from build123d import *

# Parameters (mm, degrees)
SKETCH1_R      = 3
EXTRUDE1_DEPTH = 18
SKETCH1_3_R    = 19.05
EXTRUDE2_DEPTH = 10
SKETCH2_R      = 1.52
EXTRUDE3_DEPTH = 37.59
EXTRUDE4_START = -2.6
SKETCH3_W      = 29.21
SKETCH3_H      = 15
EXTRUDE4_DEPTH = 34.99
EXTRUDE6_DEPTH = 10
SKETCH8_R      = 1.53
EXTRUDE7_DEPTH = 43
EXTRUDE8_DEPTH = 37.59


with BuildPart() as part:
    # Sketch1 → Extrude1 (new body)
    with BuildSketch(Plane(origin=(0, 0, 0), x_dir=(1, 0, 0), z_dir=(0, 1, 0))):
        with BuildLine():
            Line((-10.033035154, 21.134136258), (126.344272034, 21.134136258))
            ThreePointArc((126.344272034, 21.134136258), (129.573902971, 21.670020662), (132.457392138, 23.220239455))
            ThreePointArc((132.457392138, 23.220239455), (166.412495407, 0.194425945), (125.416806741, -1.383749149))
            ThreePointArc((125.416806741, -1.383749149), (121.751361628, 3.344530461), (116.04264662, 5.134136258))
            Line((116.04264662, 5.134136258), (0.26859026, 5.134136258))
            ThreePointArc((0.26859026, 5.134136258), (-5.440124747, 3.344530461), (-9.10556986, -1.383749149))
            ThreePointArc((-9.10556986, -1.383749149), (-50.101258526, 0.194425945), (-16.146155257, 23.220239455))
            ThreePointArc((-16.146155257, 23.220239455), (-13.262666091, 21.670020662), (-10.033035154, 21.134136258))
        make_face()
        with Locations((-29.34438156, 6.134136258)):
            Circle(SKETCH1_R, mode=Mode.SUBTRACT)
        with Locations((145.65561844, 6.134136258)):
            Circle(SKETCH1_R, mode=Mode.SUBTRACT)
    extrude(amount=EXTRUDE1_DEPTH)

    # Sketch1<3> → Extrude2 (cut)
    with BuildSketch(Plane(origin=(0, 0, 0), x_dir=(1, 0, 0), z_dir=(0, 1, 0))):
        with Locations((-29.34438156, 6.134136258)):
            Circle(SKETCH1_3_R)
        with Locations((145.65561844, 6.134136258)):
            Circle(SKETCH1_3_R)
    extrude(amount=EXTRUDE2_DEPTH, mode=Mode.SUBTRACT)

    # Sketch2 → Extrude3 (cut, through all)
    with BuildSketch(Plane(origin=(0, 0, -21.134136258), x_dir=(-1, 0, 0), z_dir=(0, 0, -1))):
        with Locations((-68.542401875, 7.04)):
            Circle(SKETCH2_R)
        with Locations((-47.61061844, 7.04)):
            Circle(SKETCH2_R)
    extrude(amount=-EXTRUDE3_DEPTH, mode=Mode.SUBTRACT)

    # Sketch3 → Extrude4 (cut, through all)
    with BuildSketch(Plane(origin=(0, 0, -21.134136258), x_dir=(-1, 0, 0), z_dir=(0, 0, -1)).offset(EXTRUDE4_START)):
        with Locations((-58.15561844, 7.5)):
            Rectangle(SKETCH3_W, SKETCH3_H)
    extrude(amount=-EXTRUDE4_DEPTH, mode=Mode.SUBTRACT)

    # Sketch6 → Extrude6 (cut)
    with BuildSketch(Plane(origin=(0, 18, 0), x_dir=(1, 0, 0), z_dir=(0, 1, 0))):
        with BuildLine():
            Line((41.01061844, 13.134136258), (41.01061844, 16.546636258))
            ThreePointArc((41.01061844, 16.546636258), (40.545650455, 17.669168273), (39.42311844, 18.134136258))
            Line((39.42311844, 18.134136258), (4.59811844, 18.134136258))
            ThreePointArc((4.59811844, 18.134136258), (3.475586425, 17.669168273), (3.01061844, 16.546636258))
            Line((3.01061844, 16.546636258), (3.01061844, 9.721636258))
            ThreePointArc((3.01061844, 9.721636258), (3.475586425, 8.599104243), (4.59811844, 8.134136258))
            Line((4.59811844, 8.134136258), (39.42311844, 8.134136258))
            ThreePointArc((39.42311844, 8.134136258), (40.545650455, 8.599104243), (41.01061844, 9.721636258))
            Line((41.01061844, 9.721636258), (41.01061844, 13.134136258))
        make_face()
        with BuildLine():
            Line((75.30061844, 9.721636258), (75.30061844, 13.134136258))
            Line((75.30061844, 13.134136258), (75.30061844, 16.546636258))
            ThreePointArc((75.30061844, 16.546636258), (75.765586425, 17.669168273), (76.88811844, 18.134136258))
            Line((76.88811844, 18.134136258), (111.71311844, 18.134136258))
            ThreePointArc((111.71311844, 18.134136258), (112.835650455, 17.669168273), (113.30061844, 16.546636258))
            Line((113.30061844, 16.546636258), (113.30061844, 9.721636258))
            ThreePointArc((113.30061844, 9.721636258), (112.835650455, 8.599104243), (111.71311844, 8.134136258))
            Line((111.71311844, 8.134136258), (76.88811844, 8.134136258))
            ThreePointArc((76.88811844, 8.134136258), (75.765586425, 8.599104243), (75.30061844, 9.721636258))
        make_face()
    extrude(amount=-EXTRUDE6_DEPTH, mode=Mode.SUBTRACT)

    # Sketch8 → Extrude7 (cut)
    with BuildSketch(Plane(origin=(75.30061844, 0, 0), x_dir=(0, 0, -1), z_dir=(1, 0, 0))):
        with Locations((13.696636258, 12.37)):
            Circle(SKETCH8_R)
    extrude(amount=-EXTRUDE7_DEPTH, mode=Mode.SUBTRACT)

    # Sketch9 → Extrude8 (cut, through all)
    with BuildSketch(Plane(origin=(0, 0, -21.134136258), x_dir=(-1, 0, 0), z_dir=(0, 0, -1))):
        with BuildLine():
            ThreePointArc((-68.427924828, 0), (-58.131552552, -10.4619369), (-47.724510158, -0.110083234))
            ThreePointArc((-47.724510158, -0.110083234), (-47.724656491, -0.055040839), (-47.725095487, 0))
            Line((-47.725095487, 0), (-68.427924828, 0))
        make_face()
        with BuildLine():
            Line((-68.427924828, 0), (-47.725095487, 0))
            ThreePointArc((-47.725095487, 0), (-58.076510158, 10.241916766), (-68.427924828, 0))
        make_face()
    extrude(amount=-EXTRUDE8_DEPTH, mode=Mode.SUBTRACT)


solid = part.part
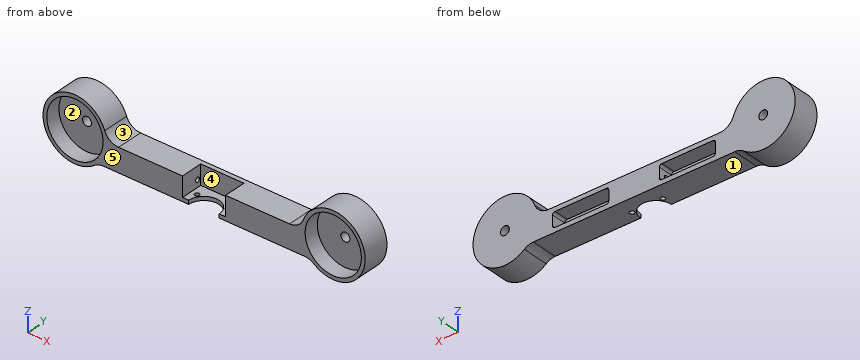
Can you work these out from the model? Positions are in its coordinate system, mm. Face numbers are marked on the shaded views. A direction names the side the tool comes from. Round coordinates to 2 decimals unless told otherwise and drop trailing zeros. Write each loop counter-clockwise with the first axis right and the second up, starting at its lowest first coordinate (ties: lowest second). Pieces come first, ordered by that corner, then holes. Notation, with made-up numbers: (82, 77) -> (124, 77) arc R31 cw to (124, 113) -> close; hole circle Ø3 at (20, 63.25). An arc over 180 degrees is marked (long way). One line per question, with ' | ' between items. Start each with the question number.
1) On a 3-axis mill with a long thin cutter (end or side, diameter ignored), from which of +Z, -Z, +X, -X, +Y, -Y can I reach the whole of each face in a straight line? I mean the marked faces 1, 2 and 3. Say none if no direction works.
2) Suppose I cut it at D-D on x = 58.5. Write out the boundary of the cut face in (y, z).
3) I need wall thicknesses on line 1 (Z direction, x = 102, y = 10.5); line 2 (Z direction, x = 145.5, y = 15.5); line 3 (X direction, y = 4.75, z = 5.5). Which ranges of each line are inside material? Lowest first, please. Write a range as [from, to].
4) Suppose I cut it at C-C on x = 130. Write out the boundary of the cut face in (y, z).
5) If we mould it in two halves opening along X, with no side actions, what happens to the marked faces 4 and 5? For each: released by +X, released by -X, zero draft, split by the parting line, or undercut.
6) Suppose I cut it at A-A on y = 2. Write out the boundary of the cut face in (x, z).
7) Suppose I cut it at B-B on z = 5. Write out the boundary of the cut face in (x, y).
8) I'm going to push flat-ended pins straight in: P1, Ø5, axis at y = 13.5, z = 6, coming from the +X side; P2, Ø10, axis at x = 59.5, y = 2, coming from the +Z side; P3, Ø4, axis at x = 68.54, y = 7.04, coming from the +Z side; P4, Ø5, axis at x = 23.5, z = -13, coming from the +Y side. Where does each tip first touch, or does it pass through?
Return value:
1) face 1: -Z, +Y, -Y | face 2: -Y | face 3: +Z, +Y, -Y
2) outline: (10.23, -21.13) -> (18, -21.13) -> (18, -5.13) -> (15, -5.13) -> (15, -18.53) -> (10.23, -18.53) -> close
3) line 1: z = [-21.13, -18.13], [-8.13, -5.13] | line 2: z = [-27.72, -9.13], [-3.14, 15.46] | line 3: x = [-47.53, -44.43], [-14.26, -11.16], [127.47, 130.57], [160.74, 163.84]
4) outline: (0, -21.83) -> (18, -21.83) -> (18, 8.73) -> (0, 8.73) -> (0, 4.72) -> (10, 4.72) -> (10, -16.99) -> (0, -16.99) -> close
5) face 4: undercut | face 5: zero draft
6) outline: (-16.15, -23.22) arc R10 cw to (-10.03, -21.13) -> (47.94, -21.13) -> (47.94, -18.53) -> (43.55, -18.53) -> (43.55, -5.13) -> (0.27, -5.13) arc R10 cw to (-9.11, 1.38) arc R21.59 ccw (long way) to start; (68.21, -21.13) -> (126.34, -21.13) arc R10 cw to (132.46, -23.22) arc R21.59 ccw (long way) to (125.42, 1.38) arc R10 cw to (116.04, -5.13) -> (72.76, -5.13) -> (72.76, -18.53) -> (68.21, -18.53) -> close; hole circle Ø38.1 at (-29.34, -6.13); hole circle Ø38.1 at (145.66, -6.13)
7) outline: (-47.84, 0) -> (-44.8, 0) -> (-44.8, 10) -> (-13.89, 10) -> (-13.89, 0) -> (-10.85, 0) -> (-10.85, 18) -> (-47.84, 18) -> close; (127.16, 0) -> (130.2, 0) -> (130.2, 10) -> (161.11, 10) -> (161.11, 0) -> (164.15, 0) -> (164.15, 18) -> (127.16, 18) -> close
8) P1: stops at x = 164.98 | P2: passes through | P3: stops at z = -18.53 | P4: stops at y = 8
